from build123d import *

# Parameters (mm, degrees)
F0_W     = 55
F0_H     = 130
F1_DEPTH = 3
F3_D     = 3
F4_SIZE  = 50


with BuildPart() as f1:
    # F0 (on Top) → F1 (new body)
    with BuildSketch(Plane.XY):
        with Locations((27.5, 65)):
            Rectangle(F0_W, F0_H)
    extrude(amount=F1_DEPTH)

    # F3 (through all)
    with Locations(Plane.XY.offset(3)):
        with Locations((25, 25), (25, 65)):
            Hole(F3_D / 2)

    # F4
    f4_edges = [f1.edges().sort_by_distance(p)[0] for p in [
        (55, 130, 1.5),
    ]]
    chamfer(f4_edges, length=F4_SIZE)

    # F5: F1 across plane


with BuildPart() as f1_1:
    add(f1.part)
    add(f1.part.mirror(Plane.YZ))


solid = f1_1.part
Source: CAD feature listing. Evaluate the final solid. Frame: model axes, mm. Round coordinates to 2 decimals unless told otherwise and drop trailing zeros. Loops run counter-clockwise (first coordinate to the right, second up) from the corner with the lowest first, then second, coordinate; pieces in that order, holes last. Notation, with made-up numbers: (-5.75, 7.25) - (44.25, 7.25) arc R7 ccw to (44.25, 12.25) - close; hole circle Ø2 at (-7, -27). An arc over 180 degrees is marked (long way). Write item = value, one per line. Start each with the question number.
Item 1: Section query A-A on y = 65. Output: boundary loops of the cut face in (x, z), plus the area to 3 significant figures.
Item 2: Mould query, pull axis Y, two halves, no side actions, for faces 1 (the face through (26.11, 26.01, 1.48)), 2 (the face through (55, 39, 1)), 3 (the face through (1, 0, 1)). Classes: released by +Y, released by -Y, zero draft, split by the parting line, or undercut.
Item 3: Section query B-B on x = -25. Output: boundary loops of the cut face in (y, z), plus the area to 3 significant figures.
Item 4: Section query C-C on z = 2.55. Output: boundary loops of the cut face in (x, y), plus the area to 3 significant figures.
Item 5: Material intervals for line 1 (Y direction, x = 24, z = 2.45); line 2 (X direction, y = 65, z = 0.85); line 3 (Y direction, x = 25, z = 0.7), sorted ascending.
Item 6: Section query D-D on y = 93. Output: boundary loops of the cut face in (x, z), plus the area to 3 significant figures.
Results list:
q1.outline = (-55, 0) - (-26.5, 0) - (-26.5, 3) - (-55, 3) - close; (-23.5, 0) - (23.5, 0) - (23.5, 3) - (-23.5, 3) - close; (26.5, 0) - (55, 0) - (55, 3) - (26.5, 3) - close
q1.area = 312 mm²
q2.face_1 = undercut
q2.face_2 = zero draft
q2.face_3 = released by -Y
q3.outline = (0, 0) - (23.5, 0) - (23.5, 3) - (0, 3) - close; (26.5, 0) - (63.5, 0) - (63.5, 3) - (26.5, 3) - close; (66.5, 0) - (110, 0) - (110, 3) - (66.5, 3) - close
q3.area = 312 mm²
q4.outline = (-55, 0) - (55, 0) - (55, 80) - (5, 130) - (-5, 130) - (-55, 80) - close; hole circle Ø3 at (-25, 25); hole circle Ø3 at (-25, 65); hole circle Ø3 at (25, 25); hole circle Ø3 at (25, 65)
q4.area = 11,800 mm²
q5.line_1 = 0 to 23.88, 26.12 to 63.88, 66.12 to 111
q5.line_2 = -55 to -26.5, -23.5 to 23.5, 26.5 to 55
q5.line_3 = 0 to 23.5, 26.5 to 63.5, 66.5 to 110
q6.outline = (-42, 0) - (42, 0) - (42, 3) - (-42, 3) - close
q6.area = 252 mm²
